Model file for the job. Use its own axes, mm. Face numbers are marked on the shaded views. A direction names the side the tool comes from. Round coordinates to 2 decimals unless told otherwise and drop trailing zeros. Loops run counter-clockwise (first coordinate to the right, second up) from the corner with the lowest first, then second, coordinate; pieces in that order, holes last. Notation, with made-up numbers: M 43,5.25 L 86,5.25 A24 ccw 86,38.25 Z; hole C -5.75,-7.75 d2. An arc over 180 degrees is marked long. Use a Markdown table: item, result. Add a question column.
Q1. Cut at A-A (y = 0). Give the cut face in (x, z) (3 decimals).
Q2. Probe line 1 (X direction, y = -1.9, z = 0.3) (3 decimals); line 2 (Z direction, x = 6.5, y = -0.9); line 3 (Z direction, x = 6.75, y = -0.05). List the from-to ranges inside material, lowest first. Write a range as from..to.
Q3. Tool access for the marked faces 1, 2 and 3: list every direction of +Z, -Z, +X, -X, +Y, -Y with a clear straight run to the whole face (end or side of a thin tool).
Q4. Cut at D-D (x = 4.75). Give the cut face in (y, z).
Q5. Cut at C-C (x = 3.5). Give the cut face in (y, z), plus the area to 3 significant figures.
Q6. Pin check, flat tips, straight feed: pin 1 (1.5 mm diameter, centred on x = 1, z = 2, fed in from -Y); pin 2 (2 mm diameter, centred on x = 6.5, y = -1, fed in from -Z); pin 3 (1.5 mm diameter, centred on y = 1.5, z = -2, fed in from -X). Stop position of each tip, or through.
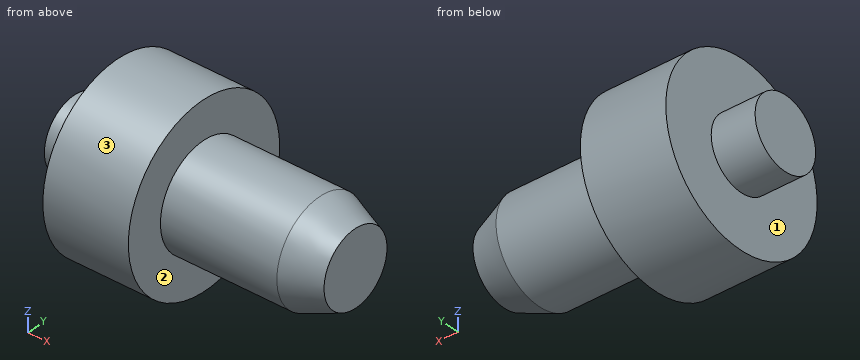
Autodesk Inventor part; units mm, degrees
ref_plane "YZ Plane" through (0, 0, 0) normal (1, 0, 0) x (0, 1, 0)
ref_plane "XZ Plane" through (0, 0, 0) normal (0, 1, 0) x (-1, 0, 0)
ref_plane "XY Plane" through (0, 0, 0) normal (0, 0, 1) x (1, 0, 0)
sketch "Sketch1" plane through (0, 0, 0) normal (0, 0, 1) x (1, 0, 0)
  line L0 (0, 0) -> (1.25, 0)
  line L1 (1.25, 0) -> (1.25, 1)
  line L2 (1.25, 1) -> (0, 1)
  line L3 (0, 1) -> (0, 0)
  line L4 (1.25, 0) -> (3.685, 0)
  line L5 (3.685, 0) -> (3.685, 2.5)
  line L6 (3.685, 2.5) -> (1.25, 2.5)
  line L7 (1.25, 2.5) -> (1.25, 0)
  line L8 (3.685, 0) -> (8, 0)
  line L9 (8, 0) -> (8, 1.44)
  line L10 (8, 1.44) -> (3.685, 1.44)
  line L11 (3.685, 1.44) -> (3.685, 0)
  dimension "d0" = 1.25
  dimension "d1" = 3.685
  dimension "d2" = 8
  dimension "d3" = 2
  dimension "d4" = 5
  dimension "d5" = 2.88
revolve "Revolution1" add sketch "Sketch1" angle 360 about axis through (3.685, 0, 0) along (1, 0, 0)
chamfer "Chamfer1" distance 0.4 distance2 1 1 edges at (8, -1.44, 0) measured on face at (8, -0.2568, -0.5255)
properties part number "403-04" material "Brass, Soft Yellow"
Checked values:
| question | item | result |
|---|---|---|
| 1 | outline | M 0,-1 L 1.25,-1 L 1.25,-2.5 L 3.685,-2.5 L 3.685,-1.44 L 7,-1.44 L 8,-1.04 L 8,1.04 L 7,1.44 L 3.685,1.44 L 3.685,2.5 L 1.25,2.5 L 1.25,1 L 0,1 Z |
| 2 | line 1 | x = 1.25..3.685 |
| 2 | line 2 | z = -1.12..1.12 |
| 2 | line 3 | z = -1.44..1.44 |
| 3 | face 1 | -X |
| 3 | face 2 | +X |
| 3 | face 3 | +X, -X |
| 4 | outline | C 0,0 d2.88 |
| 5 | outline | C 0,0 d5 |
| 5 | area | 19.6 mm^2 |
| 6 | pin 1 | stops at y = -2.14 |
| 6 | pin 2 | stops at z = -1.44 |
| 6 | pin 3 | stops at x = 1.25 |
